from build123d import *

# Parameters (mm, degrees)
SKETCH1_R           = 2
BOSS_EXTRUDE1_DEPTH = 36
CUT_EXTRUDE1_START  = -5
CUT_EXTRUDE1_DEPTH  = 5
CUT_EXTRUDE2_DEPTH  = 5


with BuildPart() as part:
    # Sketch1 → Boss-Extrude1 (new body)
    with BuildSketch(Plane.XY):
        Circle(SKETCH1_R)
    extrude(amount=BOSS_EXTRUDE1_DEPTH)

    # Sketch2 → Cut-Extrude1 (cut)
    with BuildSketch(Plane.XY.offset(36).offset(CUT_EXTRUDE1_START)):
        with BuildLine():
            Line((-1.732050808, -1), (1.732050808, -1))
            ThreePointArc((1.732050808, -1), (0, -2), (-1.732050808, -1))
        make_face()
    extrude(amount=CUT_EXTRUDE1_DEPTH, mode=Mode.SUBTRACT)

    # Sketch3 → Cut-Extrude2 (cut)
    with BuildSketch(Plane(origin=(0, 0, 5), x_dir=(-1, 0, 0), z_dir=(0, 0, -1))):
        with BuildLine():
            Line((1.732050808, -1), (-1.732050808, -1))
            ThreePointArc((-1.732050808, -1), (0, -2), (1.732050808, -1))
        make_face()
    extrude(amount=-CUT_EXTRUDE2_DEPTH, mode=Mode.SUBTRACT)


solid = part.part
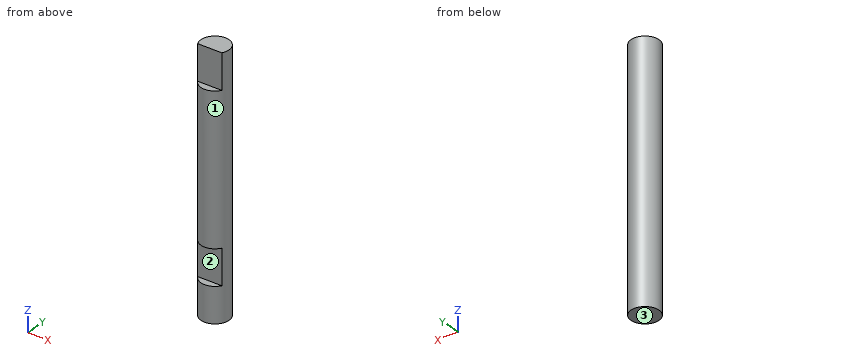
The listing builds one solid part. Answer for the finished solid, in the listing's coordinates (mm). Face numbers are marked on the shaded views. Round coordinates to 2 decimals unless told otherwise and drop trailing zeros. Write each loop counter-clockwise with the first axis right and the second up, starting at its lowest first coordinate (ties: lowest second). Pieces come first, ordered by that corner, then holes. Notation, with made-up numbers: M 32.25,88.25 L 61.25,88.25 A14 ccw 61.25,101.25 Z; hole C 75.5,-27.5 d6. An arc over 180 degrees is marked long. Write each question's results on one line, items separated by ' | '. Start each with the question number.
Item 1: The mould has two halves that part along Z. Classify the marked faces 1, 2 and 3: +Z half, -Z half, draft (parallel to the pull), parting line (faces both ways), or undercut.
Item 2: Find section C-C on z = 18.5. Write down the section's boundary in (x, y).
Item 3: Find section B-B on y = 1.2. Write down the section's boundary in (x, z), and give its area (3 significant figures).
Item 4: Find section D-D on x = 0.55. Write down the section's boundary in (y, z), and give its area (3 significant figures).
Item 5: Straight lines are drawn through the part: probe 1 along Z at (x, y) = (1.35, -1.1); probe 2 along Y at (x, z) = (1, 17); probe 3 along X at (y, z) = (-0.3, 15). For each, find the intervals that lie inside material, in ascending order.
Item 6: Find section A-A on x = -1. Write down the section's boundary in (y, z), and give its area (3 significant figures).
Item 7: Given pin 1 Ø0.5 at (x, y) = (-1, -1.5) entering from +Z; pin 2 Ø0.5 at (x, y) = (-1, -1.5) entering from -Z; pin 3 Ø1 at (x, z) = (1.5, 6.5) entering from +Y; pin 4 Ø1 at (y, z) = (-1.5, 29.5) entering from -X, each flat-ended and moving along its own axis, determine where each tip first touches the part or whether it passes through.
Answer block:
1) face 1: draft | face 2: undercut | face 3: -Z half
2) outline: C 0,0 d4
3) outline: M -1.6,0 L 1.6,0 L 1.6,36 L -1.6,36 Z | area: 115 mm²
4) outline: M -1.92,0 L 1.92,0 L 1.92,36 L -1,36 L -1,31 L -1.92,31 L -1.92,10 L -1,10 L -1,5 L -1.92,5 Z | area: 129 mm²
5) probe 1: z = 0 to 5, 10 to 31 | probe 2: y = -1.73 to 1.73 | probe 3: x = -1.98 to 1.98
6) outline: M -1.73,0 L 1.73,0 L 1.73,36 L -1,36 L -1,31 L -1.73,31 L -1.73,10 L -1,10 L -1,5 L -1.73,5 Z | area: 117 mm²
7) pin 1: stops at z = 31 | pin 2: stops at z = 0 | pin 3: stops at y = 1.73 | pin 4: stops at x = -1.73
